Source: CAD feature listing. Evaluate the final solid. Frame: model axes, mm. A direction names the side the tool comes from. Coordinates: 2 decimals unless noted, no trailing zeros. Loops run counter-clockwise (first coordinate to the right, second up) from the corner with the lowest first, then second, coordinate; pieces in that order, holes last. Notation, with made-up numbers: (-33.75, 76.5) -> (-24.75, 76.5) arc R33 cw to (-24.75, 108.5) -> close; hole circle Ø1 at (57.25, 60.25). An arc over 180 degrees is marked (long way). Answer as CSV lines item,"result".
from build123d import *

# Parameters (mm, degrees)
SKETCH2_W            = 540
SKETCH2_H            = 120
BOSS_EXTRUDE1_DEPTH  = 3.175
SKETCH3_W            = 60
SKETCH3_H            = 20
CUT_EXTRUDE1_DEPTH   = 554.181779007
FILLET1_R            = 10
FILLET2_R            = 10
M5_CLEARANCE_HOLE1_D = 5.8
LPATTERN1_COUNT      = 4
LPATTERN1_PITCH      = 119.5
SKETCH6_R            = 11
SKETCH6_W            = 29
SKETCH6_H            = 55
CUT_EXTRUDE2_DEPTH   = 518.960257277
FILLET3_R            = 3.175


with BuildPart() as part:
    # Sketch2 → Boss-Extrude1 (new body)
    with BuildSketch(Plane.XY):
        with Locations((270, 60)):
            Rectangle(SKETCH2_W, SKETCH2_H)
    extrude(amount=BOSS_EXTRUDE1_DEPTH)

    # Sketch3 → Cut-Extrude1 (cut, through all)
    with BuildSketch(Plane.XY.offset(3.175)):
        with BuildLine():
            Line((0, 0), (61, 0))
            Line((61, 0), (61, 31))
            Line((61, 31), (39.071067812, 52.928932188))
            ThreePointArc((39.071067812, 52.928932188), (36.142135624, 60), (39.071067812, 67.071067812))
            Line((39.071067812, 67.071067812), (61, 89))
            Line((61, 89), (61, 120))
            Line((61, 120), (0, 120))
            Line((0, 120), (0, 0))
        make_face()
        with BuildLine():
            Line((479, 89), (479, 120))
            Line((479, 120), (540, 120))
            Line((540, 120), (540, 0))
            Line((540, 0), (479, 0))
            Line((479, 0), (479, 31))
            Line((479, 31), (500.928932188, 52.928932188))
            ThreePointArc((500.928932188, 52.928932188), (503.857864376, 60), (500.928932188, 67.071067812))
            Line((500.928932188, 67.071067812), (479, 89))
        make_face()
        with Locations((270, 110)):
            Rectangle(SKETCH3_W, SKETCH3_H)
        with Locations((150.5, 110)):
            Rectangle(SKETCH3_W, SKETCH3_H)
        with Locations((389.5, 110)):
            Rectangle(SKETCH3_W, SKETCH3_H)
    extrude(amount=-CUT_EXTRUDE1_DEPTH, mode=Mode.SUBTRACT)

    # Fillet1
    fillet1_edges = [part.edges().sort_by_distance(p)[0] for p in [
        (61, 89, 1.5875),
        (61, 31, 1.5875),
        (479, 31, 1.5875),
        (479, 89, 1.5875),
    ]]
    fillet(fillet1_edges, radius=FILLET1_R)

    # Fillet2
    fillet2_edges = [part.edges().sort_by_distance(p)[0] for p in [
        (419.5, 100, 1.5875),
        (359.5, 100, 1.5875),
        (300, 100, 1.5875),
        (240, 100, 1.5875),
        (180.5, 100, 1.5875),
        (120.5, 100, 1.5875),
    ]]
    fillet(fillet2_edges, radius=FILLET2_R)
    fillet2_2_edges = [part.edges().sort_by_distance(p)[0] for p in [
        (419.5, 120, 1.5875),
        (359.5, 120, 1.5875),
        (300, 120, 1.5875),
        (240, 120, 1.5875),
        (180.5, 120, 1.5875),
        (120.5, 120, 1.5875),
    ]]
    fillet(fillet2_2_edges, radius=FILLET2_R - 0.0001)  # a hair under: the kernel refuses the full size

    # M5 Clearance Hole1 (through all)
    with Locations(Plane(origin=(90.75, 10, 3.175), x_dir=(1, 0, 0), z_dir=(0, 0, 1))):
        with Locations((0, 0), (0, 100)):
            m5_clearance_hole1 = Hole(M5_CLEARANCE_HOLE1_D / 2)

    # LPattern1: M5 Clearance Hole1 ×4
    with Locations(*[(i * LPATTERN1_PITCH, 0, 0) for i in range(1, LPATTERN1_COUNT)]):
        add(m5_clearance_hole1, mode=Mode.SUBTRACT)

    # Sketch6 → Cut-Extrude2 (cut, through all)
    with BuildSketch(Plane.XY.offset(3.175)):
        with Locations((160, 60)):
            Circle(SKETCH6_R)
        with Locations((210, 60)):
            Circle(SKETCH6_R)
        with Locations((95.5, 60)):
            Rectangle(SKETCH6_W, SKETCH6_H)
    extrude(amount=-CUT_EXTRUDE2_DEPTH, mode=Mode.SUBTRACT)

    # Fillet3
    fillet3_edges = [part.edges().sort_by_distance(p)[0] for p in [
        (81, 32.5, 1.5875),
        (81, 87.5, 1.5875),
        (110, 87.5, 1.5875),
        (110, 32.5, 1.5875),
    ]]
    fillet(fillet3_edges, radius=FILLET3_R)


solid = part.part
(1) Pin query (flat end, axial travel): pin 1 Ø5 at (x, y) = (90.75, 110) entering from -Z; pin 2 Ø1 at (y, z) = (52.5, 1) entering from -X. Return the tip coordinate at first contact, or that it passes through.
Computed values:
pin 1,"through"
pin 2,"x = 39"
(2) Access query for faces 4 (the flat face through (48, 76, 2)), 5 (the cylindrical face through (302.85, 116.99, 1.57)). Directions: +Z, -Z, +X, -X, +Y, -Y. A direction counts if a zero-diameter tool reaches every point of the face in a straight line with its end or side. Return the directions, or none.
Computed values:
face 4,"+Z, -Z, -X, +Y"
face 5,"+Z, -Z, +Y"
(3) Draft query along Y for faces 1 (the cylindrical face through (149, 60, 2)), 2 (the flat face through (49, 43, 2)), 3 (the flat face through (492, 76, 2)). Return one class per face: released by +Y, released by -Y, zero draft, split by the parting line, or undercut.
Computed values:
face 1,"undercut"
face 2,"released by -Y"
face 3,"released by +Y"
(4) Cut plane A-A (x = 160). Return the cut outline in (y, z) (3 decimals), then the cut area to 3 significant figures.
Computed values:
outline,"(0, 0) -> (49, 0) -> (49, 3.175) -> (0, 3.175) -> close; (71, 0) -> (100, 0) -> (100, 3.175) -> (71, 3.175) -> close"
area,"248 mm^2"
(5) Cut plane B-B (y = 22). Return the cut outline in (x, z) (3 decimals).
Computed values:
outline,"(61, 0) -> (479, 0) -> (479, 3.175) -> (61, 3.175) -> close"
(6) Cut plane C-C (z = 0.95). State how many separate pieces and enclosed holes the cut face has, then the cut area to 3 significant figures.
Computed values:
separate pieces,"1"
enclosed holes,"11"
area,"45,600 mm^2"
(7) Material intervals for L1, parallel to Y at x = 210, z = 1.05; L2, parallel to X at y = 65, z = 3; L3, parallel to Y at x = 134.5, z = 1.3, sorted ascending. Write a range as [from, to].
Computed values:
L1,"[0, 7.11], [12.89, 49], [71, 107.11], [112.89, 120]"
L2,"[37.48, 81], [110, 150.2], [169.8, 200.2], [219.8, 502.52]"
L3,"[0, 100]"
